Work out the finished part from the listing and answer in its coordinate system (mm). Round coordinates to 2 decimals unless told otherwise and drop trailing zeros. Use one line per item in the form item = value.
Autodesk Inventor part; units mm, degrees
ref_plane "РабПлоскость1" through (46.4639, 192.0462, 16) normal (-0.3670406, 0.2130535, 0.9054774) x (-0.9183225, -0.2380836, -0.3162278)
ref_plane "РабПлоскость2" through (46.4639, 0, 16) normal (0.3207767, 0.1713163, -0.9315326) x (-0.945511, 0, -0.3255902)
ref_plane "YZ Plane" through (0, 0, 0) normal (1, 0, 0) x (0, 1, 0)
sketch "Эскиз1" plane through (0, 0, 0) normal (0, 0, 1) x (1, 0, 0)
  line L0 (0, 0) -> (216, 0)
  circle A0 centre (104, 96) radius 73
  circle A1 centre (104, 96) radius 91
  line L1 (0, 180) -> (216, 236)
  line L2 (0, 87) -> (48, 0) construction
  line L3 (0, 0) -> (0, 180)
  line L4 (216, 236) -> (216, 0)
  line L5 (48, 192.4444) -> (0, 112) construction
  point P0 (43.1585, 192.0844)
  point P1 (92.1531, 205.8029)
  dimension "d2" = 146
  dimension "d3" = 182
  dimension "d6" = 236
  dimension "d7" = 180
  dimension "d8" = 96
  dimension "d15" = 48
  dimension "d16" = 48
  dimension "d17" = 87
  dimension "d18" = 68
  dimension "d22" = 216
extrude "Выдавливание2" add sketch "Эскиз1" along normal blind 12 contours A1
extrude "Выдавливание3" add sketch "Эскиз1" along normal blind 16 contours L3 L1 L4 L0
sketch "Эскиз4" plane through (0, 0, 0) normal (-1, 0, 0) x (0, 0, 1)
  line L0 (16, 180) -> (16, 0)
  point P0 (0, 0)
  point P1 (16, 87)
  point P2 (16, 112)
  dimension "d19" = 87
  dimension "d20" = 68
sketch "Эскиз5" plane through (0, 180, 16) normal (-0.2509622, 0.9679969, 0) x (0.9679969, 0.2509622, 0)
  line L0 (223.1412, 0) -> (0, 0)
  point P0 (-45.1732, 16)
  point P1 (48, 0)
  dimension "d21" = 48
ref_plane "РабПлоскость1" through (46.4639, 192.0462, 16) normal (-0.3670406, 0.2130535, 0.9054774) x (-0.9183225, -0.2380836, -0.3162278)
split "Разделение1" plane through (46.4639, 192.0462, 16) removes the side toward (-0.3670406, 0.2130535, 0.9054774)
sketch "Эскиз6" plane through (0, 0, 0) normal (0, -1, 0) x (1, 0, 0)
  line L0 (216, 16) -> (46.4639, 16)
  point P0 (0, 0)
ref_plane "РабПлоскость2" through (46.4639, 0, 16) normal (0.3207767, 0.1713163, -0.9315326) x (-0.945511, 0, -0.3255902)
split "Разделение2" plane through (46.4639, 0, 16) removes the side toward (-0.3207767, -0.1713163, 0.9315326)
chamfer "Фаска1" distance 16 angle 45 2 edges at (216, 118, 16) (131.2319, 214.0231, 16)
properties part number "Front1"
Item 1: Consider line 1 along Z through (x, y) = (194.5, 89.5); line 2 along Y through (x, z) = (44.5, 15); line 3 along Y through (x, z) = (54.5, 1). Determine where each line is inside the solid, lowest interval first.
Findings:
line_1 = 0 to 12
line_2 = 0 to 27.15, 164.85 to 176.04
line_3 = 0 to 42.35, 149.65 to 193.1
Item 2: Flat-ended cylindrical pins translate along their axes: P1, Ø4, axis at y = 59.5, z = 11, coming from the +X side; P2, Ø1.5, axis at y = 39, z = 11.5, coming from the +X side; P3, Ø10, axis at x = 150.5, y = 164.5, coming from the +Z side. Find the tip coordinate at first contact, or state that the pin passes through.
Findings:
P1 = 207
P2 = 205.25
P3 = 12
Item 3: Determine the mould class of faces 1 (the flat face through (36, 123, 12)), 2 (the flat face through (111.55, 200.54, 8.11)), 3 (the cylindrical face through (31.786, 151.372, 13.972)), 4 (the flat face through (196, 100, 16)) for opening direction X: released by +X, released by -X, zero draft, split by the parting line, or undercut.
Findings:
face_1 = undercut
face_2 = released by -X
face_3 = undercut
face_4 = zero draft
